```python
from build123d import *

# Parameters (mm, degrees)
F0_W     = 101.6
F0_H     = 76.2
F1_DEPTH = 25.654
F2_R     = 5.08
F3_R     = 18.139264
F4_DEPTH = 41.148


with BuildPart() as f1:
    # F0 (on Top) → F1 (new body)
    with BuildSketch(Plane.XY):
        with Locations((0.522892, 4.871118)):
            Rectangle(F0_W, F0_H)
    extrude(amount=F1_DEPTH)

    # F2
    f2_edges = [f1.edges().sort_by_distance(p)[0] for p in [
        (51.322892, 4.871118, 25.654),
    ]]
    fillet(f2_edges, radius=F2_R)

    # F3 (on Top) → F4 (join)
    with BuildSketch(Plane.XY):
        with Locations((-35.991579, -37.675709)):
            Circle(F3_R)
    extrude(amount=F4_DEPTH)


solid = f1.part
```
Geometry: final body of the model. Coordinates: model frame, mm. A direction names the side the tool comes from. Round coordinates to 2 decimals unless told otherwise and drop trailing zeros. Order: outer loops, then holes, each group sorted by start corner. A loop starts at its lowest first (then second) coordinate and runs counter-clockwise, first axis right, second up. Notation, with made-up numbers: M 6,15.5 L 64,15.5 A11 ccw 64,27.5 Z; hole C 56.5,14 d5. An arc over 180 degrees is marked long. Use one line per item in the form item = value. Start each with the question number.
Q1. Pin query (flat end, axial travel): pin 1 Ø1 at (x, z) = (-21.5, 9.5) entering from -Y; pin 2 Ø6 at (y, z) = (19, 27) entering from +X; pin 3 Ø12 at (y, z) = (-45.5, 13.5) entering from +X. Return the tip coordinate at first contact, or that it passes through.
Q2. Cut plane A-A (y = -18). Return loops of the section in (x, z).
Q3. Access query for faces 1 (the face through (-39.924, -55.384, 24.858)), 2 (the face through (0, 42.971, 13)), 3 (the face through (-50.277, 8, 13)). Directions: +Z, -Z, +X, -X, +Y, -Y. A direction counts if a zero-diameter tool reaches every point of the face in a straight line with its end or side. Return the directions, or none.
Q4. Cut plane B-B (z = 12). Return loops of the section in (x, y), and give its area (3 significant figures).
Q5. Material intervals for line 1 (Z direction, x = -28, y = -8.5); line 2 (Y direction, x = 0, z = 25); line 3 (X direction, y = -14, z = 18.5), sorted ascending. Write a range as [from, to].
Q6. Cut plane C-C (x = -25). Return loops of the section in (y, z), and give its area (3 significant figures).
Q7. Cut plane D-D (y = -29.5). Return loops of the section in (x, z).
Geometry results:
q1.pin_1 = -49.22
q1.pin_2 = 49.99
q1.pin_3 = -17.94
q2.outline = M -50.28,0 L 51.32,0 L 51.32,20.57 A5.08 ccw 46.24,25.65 L -50.28,25.65 Z
q3.face_1 = +Z
q3.face_2 = +Z, -Z, +X, -X, +Y
q3.face_3 = +Z, -Z, -X, +Y
q4.outline = M -50.28,-26.5 A18.14 ccw long -18.41,-33.23 L 51.32,-33.23 L 51.32,42.97 L -50.28,42.97 Z
q4.area = 8,430 mm^2
q5.line_1 = [0, 25.65]
q5.line_2 = [-33.23, 42.97]
q5.line_3 = [-50.28, 51.32]
q6.outline = M -52.11,0 L 42.97,0 L 42.97,25.65 L -23.25,25.65 L -23.25,41.15 L -52.11,41.15 Z
q6.area = 2,890 mm^2
q7.outline = M -52.18,0 L 51.32,0 L 51.32,20.57 A5.08 ccw 46.24,25.65 L -19.8,25.65 L -19.8,41.15 L -52.18,41.15 Z
